```python
from build123d import *

# Parameters (mm, degrees)
SKETCH1_W           = 112
SKETCH1_H           = 72
BOSS_EXTRUDE1_DEPTH = 4
SKETCH2_W           = 9.6
SKETCH2_H           = 4
BOSS_EXTRUDE2_DEPTH = 9.6
SKETCH3_R           = 1.55
CUT_EXTRUDE1_DEPTH  = 9.6
SKETCH4_R           = 1.55
CUT_EXTRUDE2_DEPTH  = 9.6
CUT_EXTRUDE4_DEPTH  = 9.6
CUT_EXTRUDE5_DEPTH  = 9.6
FILLET1_R           = 2
FILLET2_R           = 2


with BuildPart() as part:
    # Sketch1 → Boss-Extrude1 (new body)
    with BuildSketch(Plane.XY):
        with Locations((56, -36)):
            Rectangle(SKETCH1_W, SKETCH1_H)
    extrude(amount=BOSS_EXTRUDE1_DEPTH)

    # Sketch2 → Boss-Extrude2 (add)
    with BuildSketch(Plane.XY.offset(4)):
        with Locations((4.8, -70)):
            Rectangle(SKETCH2_W, SKETCH2_H)
        with Locations((107.2, -70)):
            Rectangle(SKETCH2_W, SKETCH2_H)
        with Locations((56, -70)):
            Rectangle(SKETCH2_W, SKETCH2_H)
    extrude(amount=BOSS_EXTRUDE2_DEPTH)

    # Sketch3 → Cut-Extrude1 (cut)
    with BuildSketch(Plane(origin=(0, -68, 0), x_dir=(1, 0, 0), z_dir=(0, 1, 0))):
        with Locations(Location((4.8, -8.8, 0), (0, 0, 270))):
            Circle(SKETCH3_R)
        with Locations(Location((56, -8.8, 0), (0, 0, 270))):
            Circle(SKETCH3_R)
        with Locations(Location((107.2, -8.8, 0), (0, 0, 270))):
            Circle(SKETCH3_R)
    extrude(amount=-CUT_EXTRUDE1_DEPTH, mode=Mode.SUBTRACT)

    # Sketch4 → Cut-Extrude2 (cut)
    with BuildSketch(Plane.XY.offset(4)):
        with Locations((47, -5)):
            Circle(SKETCH4_R)
        with Locations((65, -5)):
            Circle(SKETCH4_R)
        with Locations((56, -14)):
            Circle(SKETCH4_R)
    extrude(amount=-CUT_EXTRUDE2_DEPTH, mode=Mode.SUBTRACT)

    # Sketch5 → Cut-Extrude4 (cut)
    with BuildSketch(Plane.XY.offset(4)):
        Polygon((0, -68), (0, 0), (40, 0), align=None)
        Polygon((72, 0), (112, -68), (112, 0), align=None)
    extrude(amount=-CUT_EXTRUDE4_DEPTH, mode=Mode.SUBTRACT)

    # Sketch6 → Cut-Extrude5 (cut)
    with BuildSketch(Plane.XY.offset(4)):
        Polygon((9.6, -68), (44, -12), (51.2, -68), (51.2, -72), (9.6, -72), align=None)
        Polygon((102.4, -72), (102.4, -68), (68, -12), (60.8, -68), (60.8, -72), align=None)
    extrude(amount=-CUT_EXTRUDE5_DEPTH, mode=Mode.SUBTRACT)

    # Fillet1
    fillet1_edges = [part.edges().sort_by_distance(p)[0] for p in [
        (4.8, -68, 4),
        (107.2, -68, 4),
        (56, -68, 4),
    ]]
    fillet(fillet1_edges, radius=FILLET1_R)

    # Fillet2
    fillet2_edges = [part.edges().sort_by_distance(p)[0] for p in [
        (40, 0, 2),
        (72, 0, 2),
    ]]
    fillet(fillet2_edges, radius=FILLET2_R)


solid = part.part
```
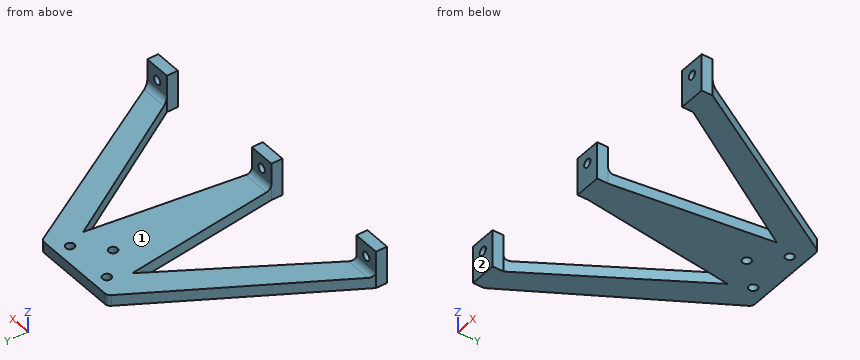
Here's how the part is built. I have some questions about the finished solid (model axes, mm). Face numbers are marked on the shaded views. A direction names the side the tool comes from. Round coordinates to 2 decimals unless told otherwise and drop trailing zeros. Write each loop counter-clockwise with the first axis right and the second up, starting at its lowest first coordinate (ties: lowest second). Pieces come first, ordered by that corner, then holes.
Q1. Please list where these lines run through material, in increasing order: probe 1 along X at (y, z) = (-70.9, 8.8); probe 2 along X at (y, z) = (-34.5, 2.5); probe 3 along X at (y, z) = (-64.5, 0.5).
Q2. Which directions (+Z, -Z, +X, -X, +Y, -Y) give clear straight access to the entire face, cutting with the end or side of a thin tool? Please do the marked faces 1 and 2.
Q3. If we section it at C-C on x = 56: Write out the boundary of the cut face in (y, z).
Q4. If we section it at D-D on y = -63.5: Write out the boundary of the cut face in (x, z).
Q5. Will these pins go through, and if not, where does the flat tip stop? P1, Ø2, axis at y = -42.5, z = 2.5, coming from the +X side; P2, Ø4.5, axis at y = -69, z = 3.5, coming from the -X side; P3, Ø3, axis at y = -53, z = 5, coming from the +X side; P4, Ø2.5, axis at x = 108, z = 11, coming from the +Y side.
Q6. If we section it at A-A on x = 107.2: Write out the boundary of the cut face in (y, z), plus the area to 3 significant figures.
Q7. If we section it at B-B on z = 11.75: Write out the boundary of the cut face in (x, y), plus the area to 3 significant figures.
Answer below:
1. probe 1: x = 0 to 3.25, 6.35 to 9.6, 51.2 to 54.45, 57.55 to 60.8, 102.4 to 105.65, 108.75 to 112
1. probe 2: x = 19.71 to 30.18, 46.89 to 65.11, 81.82 to 92.29
1. probe 3: x = 2.06 to 11.75, 50.75 to 61.25, 100.25 to 109.94
2. face 1: +Z, +X, -X, +Y
2. face 2: +Z, -Z, +X, -X, -Y
3. outline: (-72, 0) - (-15.55, 0) - (-15.55, 4) - (-66, 4) arc R2 cw to (-68, 6) - (-68, 7.25) - (-72, 7.25) - close; (-72, 10.35) - (-68, 10.35) - (-68, 13.6) - (-72, 13.6) - close; (-12.45, 0) - (0, 0) - (0, 4) - (-12.45, 4) - close
4. outline: (2.65, 0) - (12.36, 0) - (12.36, 4) - (2.65, 4) - close; (50.62, 0) - (61.38, 0) - (61.38, 4) - (50.62, 4) - close; (99.64, 0) - (109.35, 0) - (109.35, 4) - (99.64, 4) - close
5. P1: stops at x = 97.59
5. P2: stops at x = 0
5. P3: stops at x = 103.83
5. P4: stops at y = -68
6. outline: (-72, 0) - (-59.84, 0) - (-59.84, 4) - (-66, 4) arc R2 cw to (-68, 6) - (-68, 7.25) - (-72, 7.25) - close; (-72, 10.35) - (-68, 10.35) - (-68, 13.6) - (-72, 13.6) - close
6. area: 75.5 mm2
7. outline: (0, -72) - (9.6, -72) - (9.6, -68) - (0, -68) - close; (51.2, -72) - (60.8, -72) - (60.8, -68) - (51.2, -68) - close; (102.4, -72) - (112, -72) - (112, -68) - (102.4, -68) - close
7. area: 115 mm2
